from build123d import *

# Parameters (mm, degrees)
F0_W     = 9
F0_H     = 8
F0_R     = 2.53
F1_DEPTH = 26.05
F2_W     = 47.3
F2_H     = 132.3
F3_DEPTH = 22.75
F4_DEPTH = 15
F5_DEPTH = 20
F6_DEPTH = 20
F7_R     = 8.024884
F8_DEPTH = 100


with BuildPart() as f1:
    # F0 (on Top) → F1 (new body)
    with BuildSketch(Plane.XY):
        Polygon((-25.2, -67.65), (25.2, -67.65), (25.2, -12.552832), (25.2, -4), (25.2, 4), (25.2, 67.65), (-25.2, 67.65), (-25.2, 4), (-25.2, -4), align=None)
        with Locations((-29.7, 0)):
            Rectangle(F0_W, F0_H)
        with Locations((-29.7, 0)):
            Circle(F0_R, mode=Mode.SUBTRACT)
        with Locations((29.7, 0)):
            Rectangle(F0_W, F0_H)
        with Locations((29.7, 0)):
            Circle(F0_R, mode=Mode.SUBTRACT)
    extrude(amount=F1_DEPTH)

    # F2 (on Top) → F3 (cut)
    with BuildSketch(Plane.XY):
        Rectangle(F2_W, F2_H)
    extrude(amount=F3_DEPTH, mode=Mode.SUBTRACT)

    # F0 (on Top) → F4 (join)
    with BuildSketch(Plane.XY):
        with Locations((29.7, 0)):
            Rectangle(F0_W, F0_H)
        with Locations((29.7, 0)):
            Circle(F0_R, mode=Mode.SUBTRACT)
    extrude(amount=F4_DEPTH)

    # F0 (on Top) → F5 (cut)
    with BuildSketch(Plane.XY):
        with Locations((29.7, 0)):
            Rectangle(F0_W, F0_H)
        with Locations((29.7, 0)):
            Circle(F0_R, mode=Mode.SUBTRACT)
    extrude(amount=F5_DEPTH, mode=Mode.SUBTRACT)

    # F0 (on Top) → F6 (cut)
    with BuildSketch(Plane.XY):
        with Locations((-29.7, 0)):
            Rectangle(F0_W, F0_H)
        with Locations((-29.7, 0)):
            Circle(F0_R, mode=Mode.SUBTRACT)
    extrude(amount=F6_DEPTH, mode=Mode.SUBTRACT)

    # F7 (on Front) → F8 (cut)
    with BuildSketch(Plane.XZ):
        with Locations((0, 11.503653)):
            Circle(F7_R)
    extrude(amount=-F8_DEPTH, mode=Mode.SUBTRACT)


solid = f1.part
CAD build for the part. Positions are in the model's coordinates, mm. A direction names the side the tool comes from. Round coordinates to 2 decimals unless told otherwise and drop trailing zeros. Write each loop counter-clockwise with the first axis right and the second up, starting at its lowest first coordinate (ties: lowest second). Pieces come first, ordered by that corner, then holes. Notation, with made-up numbers: M 72,-34 L 78,-34 A21 ccw 78,-28 Z; hole C 23,-18 d11. An arc over 180 degrees is marked long. Put each result on its own line as item: value. Start each with the question number.
1) Saw through at A-A, the plane x = 0. Write the cut outline in (y, z), and give its area (3 significant figures).
2) Drill centre lines: probe 1 along X at (y, z) = (12, 6); probe 2 along Y at (x, z) = (-8, 4); probe 3 along Y at (x, z) = (-29.7, 22.5). Where is each one in solid material? Low to high. Write a range as [from, to].
3) Pin check, flat tips, straight feed: pin 1 Ø4 at (x, y) = (28, -0.5) entering from -Z; pin 2 Ø1.5 at (x, z) = (7, 10.5) entering from +Y; pin 3 Ø3 at (y, z) = (-3.5, 7) entering from +X; pin 4 Ø8 at (x, y) = (-29.7, 0) entering from +Z. Stop position of each tip, or through.
4) 3-axis set-ups, long thin cutter, end or side, ignore diameter. For faces 4 (the flat face through (30, -4, 23)), 5 (the flat face through (-30, 3, 20)), 6 (the flat face through (23.65, -1, 11)), 7 (the flat face through (30, 4, 23)): which of +Z, -Z, +X, -X, +Y, -Y reach the whole face in a straight line?
5) Pull direction Y, two halves, no side cores. Call faces 1 (the cylindrical face through (-1.74, 66.89, 3.67)), 2 (the flat face through (0, -66.15, 11)), 3 (the flat face through (-30, 4, 23)): pulls with the +Y half, pulls with the -Y half, needs draft (parallel to the pull), parting line crosses it, or undercut.
6) Saw through at B-B, the plane y = 0. Write the cut outline in (x, z), and give its area (3 significant figures).
7) Saw through at D-D, the plane y = -56.5. Write the cut outline in (x, z), and give its area (3 significant figures).
8) Saw through at C-C, the plane x = -11.5. Write the cut outline in (y, z).
Resolved:
1. outline: M -67.65,0 L -66.15,0 L -66.15,22.75 L 66.15,22.75 L 66.15,19.53 L 67.65,19.53 L 67.65,26.05 L -67.65,26.05 Z; M 66.15,0 L 67.65,0 L 67.65,3.48 L 66.15,3.48 Z
1. area: 491 mm²
2. probe 1: [-25.2, -23.65], [23.65, 25.2]
2. probe 2: [-67.65, -66.15], [66.15, 67.65]
2. probe 3: [-4, -2.53], [2.53, 4]
3. pin 1: z = 20
3. pin 2: y = -66.15
3. pin 3: x = 25.2
3. pin 4: z = 26.05
4. face 4: +Z, -Z, +X, -Y
4. face 5: -Z, -X, +Y, -Y
4. face 6: -Z
4. face 7: +Z, -Z, +X, +Y
5. face 1: needs draft
5. face 2: undercut
5. face 3: pulls with the +Y half
6. outline: M -34.2,20 L -32.23,20 L -32.23,26.05 L -34.2,26.05 Z; M -27.17,20 L -25.2,20 L -25.2,0 L -23.65,0 L -23.65,22.75 L 23.65,22.75 L 23.65,0 L 25.2,0 L 25.2,20 L 27.17,20 L 27.17,26.05 L -27.17,26.05 Z; M 32.23,20 L 34.2,20 L 34.2,26.05 L 32.23,26.05 Z
6. area: 285 mm²
7. outline: M -25.2,0 L -23.65,0 L -23.65,22.75 L 23.65,22.75 L 23.65,0 L 25.2,0 L 25.2,26.05 L -25.2,26.05 Z
7. area: 237 mm²
8. outline: M -67.65,0 L -66.15,0 L -66.15,22.75 L 66.15,22.75 L 66.15,0 L 67.65,0 L 67.65,26.05 L -67.65,26.05 Z
